Can you work these out from the drawing? Everything is in mm from the part's minimum corner. Give positions to 0.01 mm unless a question says otherwise; leave off trailing zeros. Order: outer loops, then holes, each group sorted by start corner. A loop starts at its lowest first (then second) coordinate and runs counter-clockwise, first axis right, second up. Notation, with made-up numbers: (73.25, 66) - (98.25, 66) arc R27 cw to (98.25, 87) - close; hole circle Ø6 at (83.25, -4.5). An arc over 180 degrees is marked (long way). Answer as a JSON object with one key per item and string values.
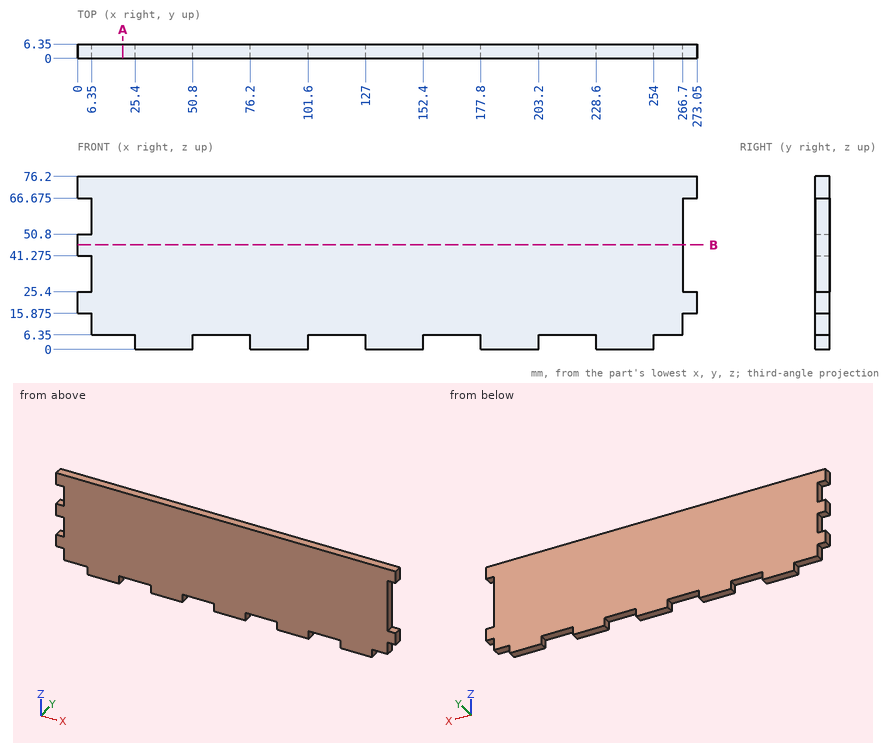
Q1. If we section it at A-A, the plane x = 20: Please give me the cut outline in (y, z), then the cut area to 3 significant figures.
Recorded:
{"outline": "(0, 6.35) - (6.35, 6.35) - (6.35, 76.2) - (0, 76.2) - close", "area": "444 mm^2"}
Q2. I need wall thicknesses on L1, parallel to X at y = 0.5, z = 26; L2, parallel to Z at x = 72, y = 5. Which ranges of each line are inside material? Lowest first, please.
Recorded:
{"L1": "x = 6.35 to 266.7", "L2": "z = 6.35 to 76.2"}
Q3. I'm going to push flat-ended pins straight in: pin 1 Ø3 at (x, y) = (172, 2.5) entering from -Z; pin 2 Ø3 at (x, y) = (243.5, 3.5) entering from -Z; pin 3 Ø1.9 at (y, z) = (4, 3) entering from +X; pin 4 Ø3 at (x, y) = (271, 3.5) entering from -Z (3 decimals). Where does each tip first touch, or does it pass through?
Recorded:
{"pin 1": "stops at z = 6.35", "pin 2": "stops at z = 0", "pin 3": "stops at x = 254", "pin 4": "stops at z = 15.875"}
Q4. If we section it at B-B, the plane z = 46: Please give me the cut outline in (x, y).
Recorded:
{"outline": "(0, 0) - (266.7, 0) - (266.7, 6.35) - (0, 6.35) - close"}
